Autodesk Inventor part; units mm, degrees
ref_plane "YZ Plane" through (0, 0, 0) normal (1, 0, 0) x (0, 1, 0)
ref_plane "XZ Plane" through (0, 0, 0) normal (0, 1, 0) x (-1, 0, 0)
ref_plane "XY Plane" through (0, 0, 0) normal (0, 0, 1) x (1, 0, 0)
sketch "Sketch1" plane through (0, 0, 0) normal (0, 0, 1) x (1, 0, 0)
  circle A0 centre (0, 0) radius 8.001
  line L0 (-0.635, 8.763) -> (0.635, 8.763)
  line L1 (0.635, 8.763) -> (0.635, 7.9758)
  line L2 (-0.635, 7.9758) -> (-0.635, 8.763)
  circle A1 centre (0, 0) radius 1.0033
  dimension "d0" = 0.762
  dimension "d2" = 0.635
  dimension "d3" = 0.635
  dimension "d4" = 16.002
  dimension "d5" = 2.0066
extrude "Extrusion1" add sketch "Sketch1" along normal mid plane 1.27 contours A0
extrude "Extrusion2" add sketch "Sketch1" along normal mid plane 1.27 contours A0 L2 L0 L1
pattern_circular "Circular Pattern1" count 16 over 360 about axis through (0, 0, 0) along (0, 0, 1) of "Extrusion2"
properties part number "Motor Gear" material "ABS Plastic"
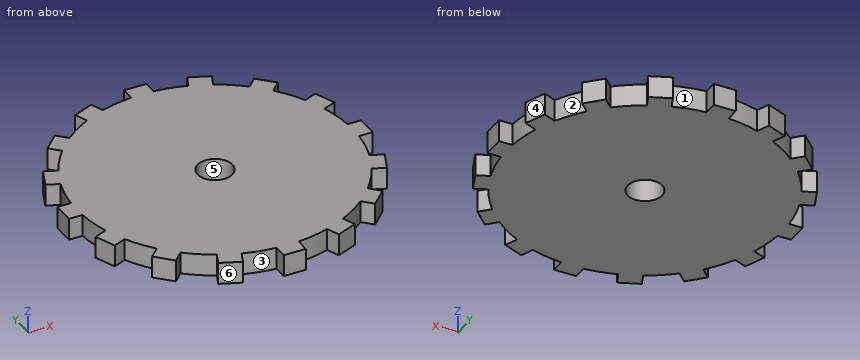
Check sheet for the modelled part. Datum: model origin and axes. Units: mm. Face numbers are marked on the shaded views. A direction names the side the tool comes from. Round coordinates to 2 decimals unless told otherwise and drop trailing zeros. Order: outer loops, then holes, each group sorted by start corner. A loop starts at its lowest first (then second) coordinate and runs counter-clockwise, first axis right, second up.
(1) Draft check along Y on the marked faces 4, 5 and 6. Enter one of: pulls with the +Y half, pulls with the -Y half, needs draft (parallel to the pull), parting line crosses it, or undercut.
(2) Access from +Z, -Z, +X, -X, +Y, -Y to the whole of each face (thin tool, end or side, straight path). Record for the marked faces 1, 2 and 3.
(3) Go/stop test with flat-tipped pins: P1, Ø0.6, axis at y = -8.5, z = -0.5, coming from the +X side; P2, Ø1.6, axis at x = 0, y = 0, coming from the -Z side; P3, Ø0.6, axis at x = -8, z = 0, coming from the +Y side; P4, Ø0.6, axis at x = 8.5, z = 0, coming from the +Y side. Record where each tip stops, or that it passes through.
(4) Cross-section at A-A, the plane y = 0. Enter the section's corners in (x, z) (3 decimals).
(5) Cross-section at C-C, the plane x = -4.25. Enter the section's corners in (y, z) (3 decimals).
(6) Cross-section at D-D, the plane y = -3. Enter the section's corners in (x, z) (3 decimals), and give its area (3 significant figures).
(7) Scan lines: probe 1 along Y at (x, z) = (0, -0.55); probe 2 along Y at (x, z) = (3.25, 0.2); probe 3 along Y at (x, z) = (1.5, -0.45). Record each from-to range of solid material in increasing order.
Check sheet entries:
1. face 4: pulls with the +Y half
1. face 5: undercut
1. face 6: pulls with the -Y half
2. face 1: +Z, -Z, +Y
2. face 2: +Z, -Z
2. face 3: +Z, -Z, -Y
3. P1: stops at x = 3.1
3. P2: passes through
3. P3: stops at y = 3.94
3. P4: stops at y = 3.1
4. outline: (-8.763, -0.635) - (-1.003, -0.635) - (-1.003, 0.635) - (-8.763, 0.635) - close; (1.003, -0.635) - (8.763, -0.635) - (8.763, 0.635) - (1.003, 0.635) - close
5. outline: (-6.779, -0.635) - (6.779, -0.635) - (6.779, 0.635) - (-6.779, 0.635) - close
6. outline: (-8.242, -0.635) - (8.242, -0.635) - (8.242, 0.635) - (-8.242, 0.635) - close
6. area: 20.9 mm2
7. probe 1: y = -8.76 to -1, 1 to 8.76
7. probe 2: y = -8.14 to 8.14
7. probe 3: y = -7.86 to 7.86
